Part model, mm, in its own coordinate system. Round coordinates to 2 decimals unless told otherwise and drop trailing zeros. Put each result on its own line as item: value. Start each with the question number.
1) Slice it at A-A on z = -1238. State how many separate pieces and enclosed holes the cut face has, then the cut area to 3 significant figures.
2) Probe line 1 along X through (y, z) = (11.6, -752.5); line 2 along X through (y, z) = (7, -654). List the from-to ranges inside material, lowest first.
3) Drop flat-ended pins along their axis: pin 1 Ø2 at (y, z) = (-2, -552) entering from -X; pin 2 Ø0.6 at (x, z) = (14, -899.5) entering from +Y; pin 3 Ø0.6 at (y, z) = (-13.5, -583.5) entering from -X. Give the stop position or say it passes through.
Autodesk Inventor part; units mm, degrees
ref_plane "C1_XY" through (0, 0, 0) normal (0, 0, 1) x (1, 0, 0)
ref_plane "C1_YZ" through (0, 0, 0) normal (1, 0, 0) x (0, 1, 0)
ref_plane "C1_ZX" through (0, 0, 0) normal (0, 1, 0) x (0, 0, 1)
sketch "Sketch_1" plane through (0, 0, 0) normal (0, 0, 1) x (1, 0, 0)
  line L0 (-15, -4) -> (-15, -13)
  arc A0 (-15, -13) -> (-13, -15) centre (-13, -13) ccw
  line L1 (-13, -15) -> (-4, -15)
  line L2 (-4, -15) -> (-4, -13)
  line L3 (-4, -13) -> (-8.25, -13)
  line L4 (-8.25, -13) -> (-8.25, -9.6642)
  line L5 (-8.25, -9.6642) -> (-4.5858, -6)
  line L6 (-4.5858, -6) -> (-0.5196, -6)
  line L7 (-0.5196, -6) -> (0, -5.7)
  line L8 (0, -5.7) -> (0.5196, -6)
  line L9 (0.5196, -6) -> (4.5858, -6)
  line L10 (4.5858, -6) -> (8.25, -9.6642)
  line L11 (8.25, -9.6642) -> (8.25, -13)
  line L12 (8.25, -13) -> (4, -13)
  line L13 (4, -13) -> (4, -15)
  line L14 (4, -15) -> (13, -15)
  arc A1 (13, -15) -> (15, -13) centre (13, -13) ccw
  line L15 (15, -13) -> (15, -4)
  line L16 (15, -4) -> (13, -4)
  line L17 (13, -4) -> (13, -8.25)
  line L18 (13, -8.25) -> (9.6642, -8.25)
  line L19 (9.6642, -8.25) -> (6, -4.5858)
  line L20 (6, -4.5858) -> (6, -0.5196)
  line L21 (6, -0.5196) -> (5.7, 0)
  line L22 (5.7, 0) -> (6, 0.5196)
  line L23 (6, 0.5196) -> (6, 4.5858)
  line L24 (6, 4.5858) -> (9.6642, 8.25)
  line L25 (9.6642, 8.25) -> (13, 8.25)
  line L26 (13, 8.25) -> (13, 4)
  line L27 (13, 4) -> (15, 4)
  line L28 (15, 4) -> (15, 13)
  arc A2 (15, 13) -> (13, 15) centre (13, 13) ccw
  line L29 (13, 15) -> (4, 15)
  line L30 (4, 15) -> (4, 13)
  line L31 (4, 13) -> (8.25, 13)
  line L32 (8.25, 13) -> (8.25, 9.6642)
  line L33 (8.25, 9.6642) -> (4.5858, 6)
  line L34 (4.5858, 6) -> (0.5196, 6)
  line L35 (0.5196, 6) -> (0, 5.7)
  line L36 (0, 5.7) -> (-0.5196, 6)
  line L37 (-0.5196, 6) -> (-4.5858, 6)
  line L38 (-4.5858, 6) -> (-8.25, 9.6642)
  line L39 (-8.25, 9.6642) -> (-8.25, 13)
  line L40 (-8.25, 13) -> (-4, 13)
  line L41 (-4, 13) -> (-4, 15)
  line L42 (-4, 15) -> (-13, 15)
  arc A3 (-13, 15) -> (-15, 13) centre (-13, 13) ccw
  line L43 (-15, 13) -> (-15, 4)
  line L44 (-15, 4) -> (-13, 4)
  line L45 (-13, 4) -> (-13, 8.25)
  line L46 (-13, 8.25) -> (-9.6642, 8.25)
  line L47 (-9.6642, 8.25) -> (-6, 4.5858)
  line L48 (-6, 4.5858) -> (-6, 0.5196)
  line L49 (-6, 0.5196) -> (-5.7, 0)
  line L50 (-5.7, 0) -> (-6, -0.5196)
  line L51 (-6, -0.5196) -> (-6, -4.5858)
  line L52 (-6, -4.5858) -> (-9.6642, -8.25)
  line L53 (-9.6642, -8.25) -> (-13, -8.25)
  line L54 (-13, -8.25) -> (-13, -4)
  line L55 (-13, -4) -> (-15, -4)
extrude "Extrusion1" add sketch "Sketch_1" against normal blind 1500
sketch "Sketch2" plane through (0, 0, -1500) normal (0, 0, -1) x (-1, 0, 0)
  point P0 (0, 0)
hole "Hole1" at (0, 0, -1500) direction (0, 0, 1) diameter 6.8 depth 1500
sketch "Sketch3" plane through (0, 0, -1500) normal (0, 0, -1) x (-1, 0, 0)
  point P0 (-11.6, 11.6)
hole "Hole2" at (11.6, 11.6, -1500) direction (0, 0, 1) diameter 4.2 depth 1500
pattern_linear "Rectangular Pattern1" count 2 spacing 23.2 along (-1, 0, 0) count 2 spacing 23.2 along (0, -1, 0) of "Hole2"
ref_plane "C1_XY" through (0, 0, 0) normal (0, 0, 1) x (1, 0, 0)
ref_plane "C1_YZ" through (0, 0, 0) normal (1, 0, 0) x (0, 1, 0)
ref_plane "C1_ZX" through (0, 0, 0) normal (0, 1, 0) x (0, 0, 1)
ref_plane "to_frame_cap1_XY" through (0, 0, 0) normal (0, 0, 1) x (1, 0, 0)
ref_plane "to_frame_cap1_YZ" through (0, 0, 0) normal (1, 0, 0) x (0, 1, 0)
ref_plane "to_frame_cap1_ZX" through (0, 0, 0) normal (0, 1, 0) x (0, 0, 1)
ref_plane "to_frame_cap2_XY" through (0, 0, -1500) normal (0, 0, -1) x (1, 0, 0)
ref_plane "to_frame_cap2_YZ" through (0, 0, -1500) normal (1, 0, 0) x (0, -1, 0)
ref_plane "to_frame_cap2_ZX" through (0, 0, -1500) normal (0, -1, 0) x (0, 0, -1)
properties part number "HFS6-3030-1500"
Recorded:
1. separate pieces: 1
1. enclosed holes: 5
1. area: 332 mm2
2. line 1: x = -15 to -13.7, -9.5 to -8.25, 8.25 to 9.5, 13.7 to 15
2. line 2: x = -15 to -13, -8.41 to -5.59, 5.59 to 8.41, 13 to 15
3. pin 1: stops at x = -6
3. pin 2: stops at y = 14.87
3. pin 3: stops at x = -14.99
